Verification items for the finished model (mm, model axes). Face numbers are marked on the shaded views. Round coordinates to 2 decimals unless told otherwise and drop trailing zeros. Write each loop counter-clockwise with the first axis right and the second up, starting at its lowest first coordinate (ties: lowest second). Pieces come first, ordered by that corner, then holes.
from build123d import *

# Parameters (mm, degrees)
BOSS_EXTRUDE1_DEPTH          = 5.5372
SKETCH6_OUTSIDE_W            = 68.81
SKETCH6_OUTSIDE_H            = 66.602
SKETCH6_OUTSIDE_R            = 6.112735428
CUT_EXTRUDE4_DEPTH           = 13.228781918
CUT_EXTRUDE4_DRAFT           = -60
MIRROR1_COPY_1_SKETCH_W      = 68.81
MIRROR1_COPY_1_SKETCH_H      = 66.602
MIRROR1_COPY_1_SKETCH_R      = 6.112735428
MIRROR1_COPY_1_DEPTH         = 13.228781918
MIRROR1_COPY_1_DRAFT         = -60
F_5_16_24_TAPPED_HOLE2_D     = 6.9088
F_5_16_24_TAPPED_HOLE2_DEPTH = 21.336
F_5_16_24_TAPPED_HOLE2_TIP   = 2.075612922


with BuildPart() as part:
    # Sketch1 → Boss-Extrude1 (new body)
    with BuildSketch(Plane.XY):
        Polygon((4.121592226, 7.1374), (-4.120373604, 7.138103572), (-8.24196583, 0.000703572), (-4.121592226, -7.1374), (4.120373604, -7.138103572), (8.24196583, -0.000703572), align=None)
    extrude(amount=BOSS_EXTRUDE1_DEPTH)


with BuildPart() as cut_extrude4_tool:
    # Sketch6 outside → Cut-Extrude4 (with draft: the straight prism first)
    with BuildSketch(Plane(origin=(0, 0, 0), x_dir=(-1, 0, 0), z_dir=(0, 0, -1))):
        Rectangle(SKETCH6_OUTSIDE_W, SKETCH6_OUTSIDE_H)
        Circle(SKETCH6_OUTSIDE_R, mode=Mode.SUBTRACT)
    extrude(amount=-CUT_EXTRUDE4_DEPTH)
    # Cut-Extrude4: the draft: its side faces are tilted about the plane it starts from
    cut_extrude4_sides = [cut_extrude4_tool.faces().sort_by_distance(p)[0] for p in [
        (0, -33.301, 6.614390959),
        (-34.405, 0, 6.614390959),
        (0, 33.301, 6.614390959),
        (34.405, 0, 6.614390959),
        (6.112735428, 0, 6.614390959),
    ]]
    draft(cut_extrude4_sides, Plane(origin=(0, 0, 0), x_dir=(-1, 0, 0), z_dir=(0, 0, -1)), CUT_EXTRUDE4_DRAFT)


with BuildPart() as part_1:
    add(part.part)

    # Cut-Extrude4: cut by cut_extrude4_tool
    add(cut_extrude4_tool.part, mode=Mode.SUBTRACT)


with BuildPart() as mirror1_copy_1_tool:
    # Mirror1 copy 1 sketch → Mirror1 copy 1 (with draft: the straight prism first)
    with BuildSketch(Plane(origin=(0, 0, 5.5372), x_dir=(-1, 0, 0), z_dir=(0, 0, 1))):
        Rectangle(MIRROR1_COPY_1_SKETCH_W, MIRROR1_COPY_1_SKETCH_H)
        Circle(MIRROR1_COPY_1_SKETCH_R, mode=Mode.SUBTRACT)
    extrude(amount=-MIRROR1_COPY_1_DEPTH)
    # Mirror1 copy 1: the draft: its side faces are tilted about the plane it starts from
    mirror1_copy_1_sides = [mirror1_copy_1_tool.faces().sort_by_distance(p)[0] for p in [
        (0, -33.301, -1.077190959),
        (-34.405, 0, -1.077190959),
        (0, 33.301, -1.077190959),
        (34.405, 0, -1.077190959),
        (6.112735428, 0, -1.077190959),
    ]]
    draft(mirror1_copy_1_sides, Plane(origin=(0, 0, 5.5372), x_dir=(-1, 0, 0), z_dir=(0, 0, 1)), MIRROR1_COPY_1_DRAFT)


with BuildPart() as part_2:
    add(part_1.part)

    # Mirror1 copy 1: cut by mirror1_copy_1_tool
    add(mirror1_copy_1_tool.part, mode=Mode.SUBTRACT)

    # 5/16-24 Tapped Hole2
    with Locations(Plane.XY.offset(5.5372)):
        with Locations((0, 0)):
            Hole(F_5_16_24_TAPPED_HOLE2_D / 2, depth=F_5_16_24_TAPPED_HOLE2_DEPTH)
            with Locations((0, 0, -(F_5_16_24_TAPPED_HOLE2_DEPTH + F_5_16_24_TAPPED_HOLE2_TIP / 2))):  # 118° drill point
                Cone(0, F_5_16_24_TAPPED_HOLE2_D / 2, F_5_16_24_TAPPED_HOLE2_TIP, mode=Mode.SUBTRACT)


solid = part_2.part
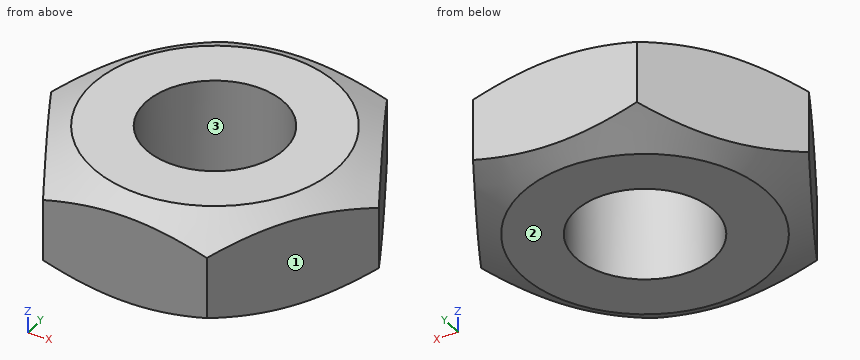
Q1. Material ranges on line 1 along Y through (x, z) = (0, 3.9); line 2 along X through (y, z) = (-0.5, 2.9); line 3 along Y through (x, z) = (2.75, 4.75), recorded low to high.
Recorded:
line 1: y = -7.14 to -3.45, 3.45 to 7.14
line 2: x = -7.95 to -3.42, 3.42 to 7.95
line 3: y = -6.95 to -2.09, 2.09 to 6.95
Q2. Depth check by flat-ended pin: P1, Ø1, axis at x = 6.5, z = 4.5, coming from the -Y side; P2, Ø6, axis at x = 0, y = 0, coming from the +Z side; P3, Ø1, axis at y = -1, z = 2, coming from the -X side. Enter the tip coordinate at first touch or a pass-through.
Recorded:
P1: stops at y = -3.88
P2: passes through
P3: stops at x = -7.95
Q3. Sectioned sample at B-B (x = 0). Enter the section's corners in (y, z), plus the area to 3 significant figures.
Recorded:
outline: (-7.14, 0.59) - (-6.11, 0) - (-3.45, 0) - (-3.45, 5.54) - (-6.11, 5.54) - (-7.14, 4.95) - close; (3.45, 0) - (6.11, 0) - (7.14, 0.59) - (7.14, 4.95) - (6.11, 5.54) - (3.45, 5.54) - close
area: 39.6 mm2
Q4. Release check for a two-part mould opening along Y. For the marked faces 1, 2 and 3 record: released by +Y, released by -Y, zero draft, split by the parting line, or undercut.
Recorded:
face 1: released by -Y
face 2: zero draft
face 3: undercut
Q5. Sectioned sample at A-A (z = 1.9). Enter the section's corners in (x, y).
Recorded:
outline: (-8.24, 0) - (-4.12, -7.14) - (4.12, -7.14) - (8.24, 0) - (4.12, 7.14) - (-4.12, 7.14) - close; hole circle Ø6.91 at (0, 0)
Q6. Sectioned sample at C-C (z = 4.7). Enter the section's corners in (x, y).
Recorded:
outline: (-7.43, -1.4) - (-4.93, -5.73) arc R7.56 ccw to (-2.5, -7.14) - (2.5, -7.14) arc R7.56 ccw to (4.93, -5.73) - (7.43, -1.4) arc R7.56 ccw to (7.43, 1.4) - (4.93, 5.73) arc R7.56 ccw to (2.5, 7.14) - (-2.5, 7.14) arc R7.56 ccw to (-4.93, 5.73) - (-7.43, 1.4) arc R7.56 ccw to start; hole circle Ø6.91 at (0, 0)
